Check sheet for the modelled part. Datum: model origin and axes. Units: mm. Face numbers are marked on the shaded views. Round coordinates to 2 decimals unless told otherwise and drop trailing zeros. Write each loop counter-clockwise with the first axis right and the second up, starting at its lowest first coordinate (ties: lowest second). Pieces come first, ordered by that corner, then holes. Notation, with made-up numbers: (-34, -33.75) - (-13, -33.75) arc R9 ccw to (-13, -18.75) - close; hole circle Ø8 at (-23.5, 37). An arc over 180 degrees is marked (long way). Answer as a JSON object with one key per item and string values. Group by question number.
Item 1: Sectioned sample at A-A on x = -9.5. Record the boundary of the cut face in (y, z).
Item 2: Gauge pin test, flat ends, axial feed: P1, Ø12, axis at x = 0.5, z = 13, coming from the -Y side; P2, Ø2, axis at x = 3, y = 0, coming from the +Z side. Record the tip position at first contact, or that the pin passes through.
Item 3: Sectioned sample at D-D on y = 4. Record the boundary of the cut face in (x, z).
Item 4: Thickness scan on line 1 (X direction, y = 7.1, z = 19.6); line 2 (Z direction, x = 9.5, y = 7.1); line 3 (Y direction, x = 15, z = 0.45). Record the ranges inside material, lowest first.
Item 5: Sectioned sample at B-B on z = 19.6. Record the boundary of the cut face in (x, y).
Item 6: Release check for a two-part mould opening along Z. For the marked faces 1, 2 and 3 record: pulls with the +Z half, pulls with the -Z half, needs draft (parallel to the pull), parting line crosses it, or undercut.
Item 7: Sectioned sample at C-C on x = -15. Record the boundary of the cut face in (y, z), plus the area to 3 significant figures.
```python
from build123d import *

# Parameters (mm, degrees)
SKETCH1_W           = 40
SKETCH1_H           = 15
BOSS_EXTRUDE1_DEPTH = 1.45
SKETCH2_W           = 40
SKETCH2_H           = 1.45
BOSS_EXTRUDE2_DEPTH = 23.55
SKETCH3_R           = 1.5
CUT_EXTRUDE1_DEPTH  = 1.45
SKETCH4_R           = 3.5
CUT_EXTRUDE2_DEPTH  = 1.45


with BuildPart() as part:
    # Sketch1 → Boss-Extrude1 (new body)
    with BuildSketch(Plane.XY):
        Rectangle(SKETCH1_W, SKETCH1_H)
    extrude(amount=BOSS_EXTRUDE1_DEPTH)

    # Sketch2 → Boss-Extrude2 (add)
    with BuildSketch(Plane.XY.offset(1.45)):
        with Locations((0, 6.775)):
            Rectangle(SKETCH2_W, SKETCH2_H)
    extrude(amount=BOSS_EXTRUDE2_DEPTH)

    # Sketch3 → Cut-Extrude1 (cut)
    with BuildSketch(Plane.XY.offset(1.45)):
        with Locations((-15, -3.5)):
            Circle(SKETCH3_R)
    cut_extrude1 = extrude(amount=-CUT_EXTRUDE1_DEPTH, mode=Mode.SUBTRACT)

    # Mirror1: Cut-Extrude1 across plane
    add(cut_extrude1.mirror(Plane(origin=(0, 0, 0), x_dir=(0, 0, 1), z_dir=(1, 0, 0))), mode=Mode.SUBTRACT)

    # Sketch4 → Cut-Extrude2 (cut)
    with BuildSketch(Plane(origin=(0, 7.5, 0), x_dir=(1, 0, 0), z_dir=(0, 1, 0))):
        with Locations((-9.5, -19.6)):
            Circle(SKETCH4_R)
    cut_extrude2 = extrude(amount=-CUT_EXTRUDE2_DEPTH, mode=Mode.SUBTRACT)

    # Mirror2: Cut-Extrude2 across plane
    add(cut_extrude2.mirror(Plane(origin=(0, 0, 0), x_dir=(0, 0, 1), z_dir=(1, 0, 0))), mode=Mode.SUBTRACT)


solid = part.part
```
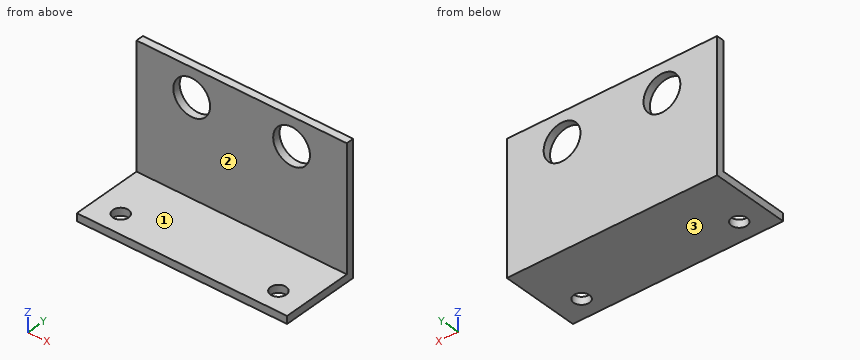
Completed:
{
 "1": {"outline": "(-7.5, 0) - (7.5, 0) - (7.5, 16.1) - (6.05, 16.1) - (6.05, 1.45) - (-7.5, 1.45) - close; (6.05, 23.1) - (7.5, 23.1) - (7.5, 25) - (6.05, 25) - close"},
 "2": {"P1": "y = 6.05", "P2": "z = 1.45"},
 "3": {"outline": "(-20, 0) - (20, 0) - (20, 1.45) - (-20, 1.45) - close"},
 "4": {"line 1": "-20 to -13, -6 to 6, 13 to 20", "line 2": "0 to 16.1, 23.1 to 25", "line 3": "-7.5 to -5, -2 to 7.5"},
 "5": {"outline": "(-20, 6.05) - (-13, 6.05) - (-13, 7.5) - (-20, 7.5) - close; (-6, 6.05) - (6, 6.05) - (6, 7.5) - (-6, 7.5) - close; (13, 6.05) - (20, 6.05) - (20, 7.5) - (13, 7.5) - close"},
 "6": {"face 1": "pulls with the +Z half", "face 2": "needs draft", "face 3": "pulls with the -Z half"},
 "7": {"outline": "(-7.5, 0) - (-5, 0) - (-5, 1.45) - (-7.5, 1.45) - close; (-2, 0) - (7.5, 0) - (7.5, 25) - (6.05, 25) - (6.05, 1.45) - (-2, 1.45) - close", "area": "51.5 mm²"}
}
